Autodesk Inventor part; units mm, degrees
ref_plane "YZ Plane" through (0, 0, 0) normal (1, 0, 0) x (0, 1, 0)
ref_plane "XZ Plane" through (0, 0, 0) normal (0, 1, 0) x (-1, 0, 0)
ref_plane "XY Plane" through (0, 0, 0) normal (0, 0, 1) x (1, 0, 0)
ref_plane "Work Plane1" through (0, 0, 0) normal (0, 0, 1) x (1, 0, 0)
sketch "Sketch1" plane through (0, 0, 0) normal (0, 0, 1) x (1, 0, 0)
  circle A0 centre (17.5, 17.5) radius 1.95
  circle A1 centre (17.5, -17.5) radius 1.95
  circle A2 centre (-17.5, -17.5) radius 1.95
  circle A3 centre (-17.5, 17.5) radius 1.95
  circle A4 centre (0, 0) radius 7.5
  line L0 (-30, 28) -> (-28, 30)
  line L1 (-30, -28) -> (-30, 28)
  line L2 (-28, -30) -> (-30, -28)
  line L3 (28, -30) -> (-28, -30)
  line L4 (30, -28) -> (28, -30)
  line L5 (30, 28) -> (30, -28)
  line L6 (28, 30) -> (30, 28)
  line L7 (-28, 30) -> (28, 30)
extrude "Extrusion1" add sketch "Sketch1" along normal blind 12 contours A0 | A1 | A2 | A3 | A4 | L0 L7 L6 L5 L4 L3 L2 L1
sketch "Sketch2" plane through (0, 0, 12) normal (0, 0, 1) x (1, 0, 0)
  point P0 (0, 0)
sketch "Sketch5" plane through (0, 0, 0) normal (0, 0, -1) x (-1, 0, 0)
  line L0 (49, -22) -> (49, -7)
  line L1 (30, -28) -> (30, 28)
  line L2 (45, 6.5) -> (45, 24.5)
  line L3 (49, -7) -> (30, -7)
  line L4 (30, -7) -> (30, -22)
  line L5 (30, -22) -> (49, -22)
  line L6 (49, -22) -> (49, -7)
  line L7 (45, 6.5) -> (30, 6.5)
  line L8 (30, 6.5) -> (30, 24.5)
  line L9 (30, 24.5) -> (45, 24.5)
  line L10 (45, 24.5) -> (45, 6.5)
  line L11 (22, 49) -> (7, 49)
  line L12 (-6.5, 45) -> (-24.5, 45)
  line L13 (7, 49) -> (7, 30)
  line L14 (7, 30) -> (22, 30)
  line L15 (22, 30) -> (22, 49)
  line L16 (22, 49) -> (7, 49)
  line L17 (-6.5, 45) -> (-6.5, 30)
  line L18 (-6.5, 30) -> (-24.5, 30)
  line L19 (-24.5, 30) -> (-24.5, 45)
  line L20 (-24.5, 45) -> (-6.5, 45)
  point P0 (0, 0)
  point P1 (-28, 30)
  dimension "d12" = 90
extrude "Extrusion4" add sketch "Sketch5" against normal up to surface (12 mm away) contours L15 L14 L13 L11 | L17 L18 L19 L12
sketch "Sketch6" plane through (24.5, 30, 0) normal (1, 0, 0) x (0, 0, -1)
  line L0 (-12, 0) -> (-12, 15)
  line L1 (0, 0) -> (-12, 0)
  line L2 (0, 0) -> (0, 15)
  line L3 (0, 15) -> (-12, 15)
  circle A0 centre (-6, 7.5) radius 3.6127
  point P0 (0, -30)
extrude "Extrusion5" cut sketch "Sketch6" against normal through all contours A0
properties part number "00_XY_stage-CHUO_SEIKI_LD-647-R1-Middle"
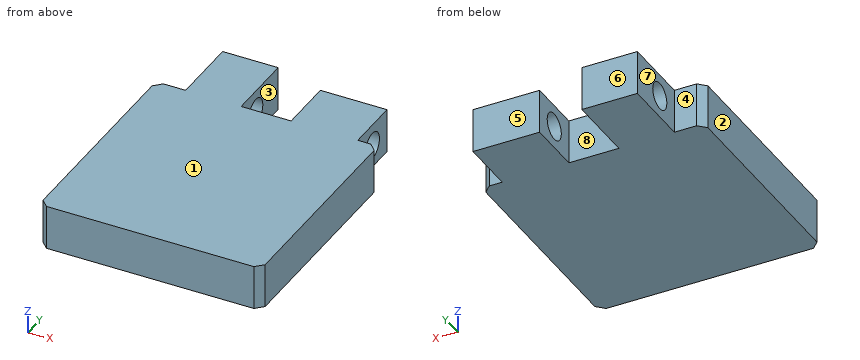
The listing builds one solid part. Answer for the finished solid, in the listing's coordinates (mm). Face numbers are marked on the shaded views. A direction names the side the tool comes from. Give positions to 0.01 mm unless a question says otherwise; leave off trailing zeros. Order: outer loops, then holes, each group sorted by start corner. A loop starts at its lowest first (then second) coordinate and runs counter-clockwise, first axis right, second up. Notation, with made-up numbers: (88.5, 42.25) - (144.5, 42.25) arc R25 ccw to (144.5, 56.25) - close; hole circle Ø10 at (36, 82.25). An arc over 180 degrees is marked (long way). Use one line per item in the form item = value.
1) Find section C-C on y = 37.5. Determine the outline of the cut face in (x, z), and give its area (3 significant figures).
Verdict:
outline = (-22, 0) - (-7, 0) - (-7, 2.39) - (-22, 2.39) - close; (-22, 9.61) - (-7, 9.61) - (-7, 12) - (-22, 12) - close; (6.5, 0) - (24.5, 0) - (24.5, 2.39) - (6.5, 2.39) - close; (6.5, 9.61) - (24.5, 9.61) - (24.5, 12) - (6.5, 12) - close
area = 158 mm^2
2) Find section D-D on z = 10.5. Determine the outline of the cut face in (x, y).
Verdict:
outline = (-30, -28) - (-28, -30) - (28, -30) - (30, -28) - (30, 28) - (28, 30) - (24.5, 30) - (24.5, 45) - (6.5, 45) - (6.5, 30) - (-7, 30) - (-7, 49) - (-22, 49) - (-22, 30) - (-28, 30) - (-30, 28) - close
3) Find section A-A on z = 6. Determine the outline of the cut face in (x, y).
Verdict:
outline = (-30, -28) - (-28, -30) - (28, -30) - (30, -28) - (30, 28) - (28, 30) - (24.5, 30) - (24.5, 33.89) - (6.5, 33.89) - (6.5, 30) - (-7, 30) - (-7, 33.89) - (-22, 33.89) - (-22, 30) - (-28, 30) - (-30, 28) - close; (-22, 41.11) - (-7, 41.11) - (-7, 49) - (-22, 49) - close; (6.5, 41.11) - (24.5, 41.11) - (24.5, 45) - (6.5, 45) - close
4) For the marked faces 1, 2, 3, 4 and 5, determine the directions among +Z, -Z, +X, -X, +Y, -Y from which every point of the face is accessible in a straight line to the end or side of a thin tool.
Verdict:
face_1 = +Z, +X, -X, +Y, -Y
face_2 = +Z, -Z, -X, +Y, -Y
face_3 = +Z, -Z, +Y
face_4 = +Z, -Z, -X, +Y
face_5 = +Z, -Z, +X, +Y
5) The mould has two halves that part along X. Classify the marked faces 6, 7 and 8: released by +X, released by -X, zero draft, split by the parting line, or undercut.
Verdict:
face_6 = zero draft
face_7 = released by -X
face_8 = undercut
6) Each of these flat-tipped pins is pushed along its axis until it touches: pin 1 (3 mm diameter, centred on x = -24.5, z = 6.5, fed in from +Y); pin 2 (6.5 mm diameter, centred on y = 37.5, z = 6, fed in from -X); pin 3 (3.5 mm diameter, centred on x = 14.5, z = 3.5, fed in from +Y). Where does it stop, or does it pass through?
Verdict:
pin_1 = 30
pin_2 = through
pin_3 = 45
7) Find section B-B on x = 22.5. Determine the outline of the cut face in (y, z).
Verdict:
outline = (-30, 0) - (45, 0) - (45, 12) - (-30, 12) - close; hole circle Ø7.23 at (37.5, 6)
8) Consider probe 1 along Y at (x, z) = (-16.25, 6); probe 2 along X at (y, z) = (39, 1.25); probe 3 along Y at (x, z) = (12, 6). Determine where each line is inside the solid, lowest interval first. Write a range as [from, to].
Verdict:
probe_1 = [-30, 33.89], [41.11, 49]
probe_2 = [-22, -7], [6.5, 24.5]
probe_3 = [-30, 33.89], [41.11, 45]
